The model under review builds one solid part; all positions refer to its coordinate system, in mm. Face numbers are marked on the shaded views. Round coordinates to 2 decimals unless told otherwise and drop trailing zeros. Order: outer loops, then holes, each group sorted by start corner. A loop starts at its lowest first (then second) coordinate and runs counter-clockwise, first axis right, second up.
Autodesk Inventor part; units mm, degrees
ref_plane "YZ Plane" through (0, 0, 0) normal (1, 0, 0) x (0, 1, 0)
ref_plane "XZ Plane" through (0, 0, 0) normal (0, 1, 0) x (-1, 0, 0)
ref_plane "XY Plane" through (0, 0, 0) normal (0, 0, 1) x (1, 0, 0)
sketch "スケッチ1" plane through (0, 0, 0) normal (1, 0, 0) x (0, 1, 0)
  circle A0 centre (0, 0) radius 28
  circle A1 centre (0, 0) radius 8
  dimension "d0" = 56
  dimension "d1" = 16
extrude "押し出し1" add sketch "スケッチ1" along normal blind 2
sketch "スケッチ2" plane through (2, 0, 0) normal (1, 0, 0) x (0, 0, -1)
  circle A0 centre (0, 0) radius 28
  line L0 (21.8575, 17.5) -> (21.8575, -17.5)
  line L1 (19.8575, -19.7403) -> (19.8575, 19.7403)
  arc A1 (21.8575, 17.5) -> (19.8575, 19.7403) centre (0, 0) ccw
  arc A2 (17.6291, -21.7535) -> (21.8575, -17.5) centre (0, 0) ccw
  arc A3 (19.8575, 19.7403) -> (17.6291, -21.7535) centre (0, 0) ccw
  arc A4 (19.8575, 16.7833) -> (19.8575, -16.7833) centre (0, 0) ccw
  dimension "d4" = 2
  dimension "d30" = 35
  dimension "d31" = 2
extrude "押し出し2" add sketch "スケッチ2" along normal blind 25 contours L0 A0 L1 | L1 A4 A0 | L1 A4
sketch "スケッチ3" plane through (27, 0, 0) normal (1, 0, 0) x (0, 0, -1)
  circle A0 centre (0, 0) radius 28
  line L0 (21.8575, -17.5) -> (21.8575, 17.5)
  line L1 (21.8575, 17.5) -> (21.8575, -17.5)
  arc A1 (21.8575, 17.5) -> (21.8575, -17.5) centre (0, 0) ccw
  arc A2 (21.8575, 14.0801) -> (21.8575, -14.0801) centre (0, 0) ccw
  line L2 (16.8575, -19.7946) -> (16.8575, 19.7946)
  dimension "d7" = 2
  dimension "d8" = 5
extrude "押し出し3" cut sketch "スケッチ3" against normal blind 25 contours L2 A2
sketch "スケッチ4" plane through (2, -17.5, -21.8575) normal (0, 0, -1) x (-1, 0, 0)
  line L0 (-25, 0) -> (-25, 35)
  line L1 (-25, 20) -> (-22, 20)
  line L2 (-22, 20) -> (-22, 15)
  line L3 (-22, 15) -> (-25, 15)
  line L4 (-25, 15) -> (-25, 20)
  line L5 (0, 35) -> (-25, 35)
  line L6 (0, 0) -> (-25, 0)
  point P0 (2, 17.5)
  dimension "d11" = 15
  dimension "d12" = 15
  dimension "d13" = 3
extrude "押し出し4" cut sketch "スケッチ4" against normal blind 25
sketch "スケッチ5" plane through (2, -17.5, -21.8575) normal (0, 0, -1) x (-1, 0, 0)
  circle A0 centre (-7, 6.5) radius 1.5
  circle A1 centre (-7, 28.5) radius 1.5
  line L0 (-13, 2.5) -> (-1, 2.5)
  line L1 (-1, 2.5) -> (-1, 32.5)
  line L2 (-1, 32.5) -> (-13, 32.5)
  line L3 (-13, 32.5) -> (-13, 2.5)
  line L4 (0, 35) -> (0, 0)
  line L5 (0, 35) -> (-25, 35)
  line L6 (0, 0) -> (-25, 0)
  point P0 (2, 17.5)
  dimension "d16" = 3
  dimension "d17" = 3
  dimension "d19" = 30
  dimension "d20" = 4
  dimension "d21" = 4
  dimension "d22" = 6
  dimension "d23" = 6
  dimension "d24" = 6
  dimension "d25" = 1
  dimension "d26" = 2.5
  dimension "d27" = 2.5
extrude "押し出し5" cut sketch "スケッチ5" against normal blind 25 contours A0 | A1
sketch "スケッチ6" plane through (2, -17.5, -21.8575) normal (0, 0, -1) x (-1, 0, 0)
  point P0 (2, 17.5)
properties part number "turn1part"
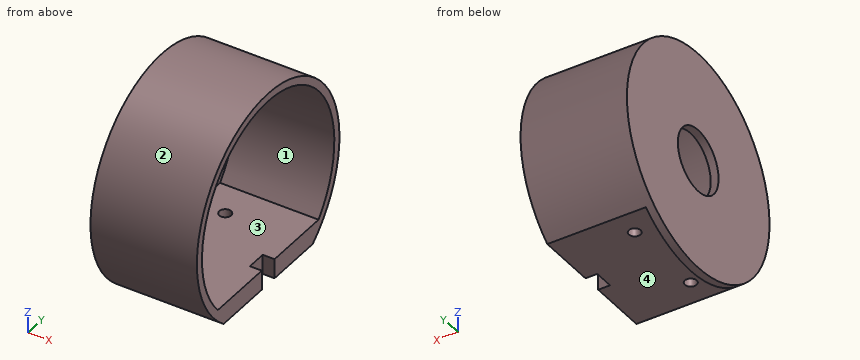
(1) Consider section B-B (z = 0). Write out the cut boundary in (x, y).
Data:
outline: (0, -28) - (27, -28) - (27, -26) - (2, -26) - (2, -8) - (0, -8) - close; (0, 8) - (2, 8) - (2, 26) - (27, 26) - (27, 28) - (0, 28) - close
(2) Insertion check: pin 1 (12 mm diameter, centred on x = 7, z = -9, fed in from +Y); pin 2 (1.5 mm diameter, centred on x = 25, z = -20.5, fed in from +Y); pin 3 (5 mm diameter, centred on x = 9, y = 11, fed in from -Z); pin 4 (12 mm diameter, centred on y = 2, z = 4.5, fed in from -X). Each pin has a flat end and moves straight along its axis. Give the tip position at first contact, or say it passes through.
Data:
pin 1: stops at y = 27.84
pin 2: stops at y = 19.85
pin 3: stops at z = -21.86
pin 4: stops at x = 0
(3) Consider section D-D (y = 21). Write out the cut boundary in (x, z).
Data:
outline: (0, -18.52) - (27, -18.52) - (27, -15.33) - (2, -15.33) - (2, 15.33) - (27, 15.33) - (27, 18.52) - (0, 18.52) - close
(4) To check wall thickness, follow probe 1 along Z at (x, y) = (18.25, 0); probe 2 along Y at (x, z) = (11, 0); probe 3 along X at (y, z) = (-16.5, 10.5). State the ranges of each line that lie inside material, in increasing order.
Data:
probe 1: z = -21.86 to -16.86, 26 to 28
probe 2: y = -28 to -26, 26 to 28
probe 3: x = 0 to 2
(5) Consider section C-C (x = 9). Write out the cut boundary in (y, z), and give its area (3 significant figures).
Data:
outline: (-19.79, -16.86) arc R26 cw (long way) to (19.79, -16.86) - (12.5, -16.86) - (12.5, -21.86) - (17.5, -21.86) arc R28 ccw (long way) to (-17.5, -21.86) - (-12.5, -21.86) - (-12.5, -16.86) - close; (-9.5, -21.86) - (9.5, -21.86) - (9.5, -16.86) - (-9.5, -16.86) - close
area: 414 mm2
(6) Consider section A-A (y = 0). Write out the cut boundary in (x, z), and give its area (3 significant figures).
Data:
outline: (0, -28) - (2, -28) - (2, -21.86) - (24, -21.86) - (24, -16.86) - (2, -16.86) - (2, -8) - (0, -8) - close; (0, 8) - (2, 8) - (2, 26) - (27, 26) - (27, 28) - (0, 28) - close
area: 240 mm2
(7) Draft analysis for pull direction Y (two halves, no side actions). For the marked faces 1, 2, 3 and 4, state which applies: pulls with the +Y half, pulls with the -Y half, needs draft (parallel to the pull), parting line crosses it, or undercut.
Data:
face 1: undercut
face 2: parting line crosses it
face 3: undercut
face 4: needs draft
